Design review of the part built by this model. Coordinates are the model's own, in mm. Face numbers are marked on the shaded views. A direction names the side the tool comes from. Give positions to 0.01 mm unless a question says otherwise; leave off trailing zeros. Loops run counter-clockwise (first coordinate to the right, second up) from the corner with the lowest first, then second, coordinate; pieces in that order, holes last. Notation, with made-up numbers: (47.5, 27.5) -> (95.5, 27.5) arc R14 ccw to (95.5, 52.5) -> close; hole circle Ø9 at (55, 13). An arc over 180 degrees is marked (long way). Use a Markdown table: item, result. Add a question column.
1. For pin 1 Ø17.5 at (x, z) = (-10, 10) entering from +Y, flat-tipped, find the tip position at first contact; note if it passes through.
2. Add section C-C (z = 32.5). State the section outline as (x, y) points (1 decimal), and give its area (3 significant figures).
3. Add section D-D (y = -3). State the section outline as (x, z) points (3 decimals), and give its area (3 significant figures).
4. For the marked faces 1 and 2, list the 3-axis set-ups (+Z, -Z, +X, -X, +Y, -Y) from which the entire face can be reached by the end or side of a thin tool; tool diameter is ignored.
5. Add section B-B (y = 11). State the section outline as (x, z) points (3 decimals).
6. Add section A-A (z = 17.5). State the section outline as (x, y) points (1 decimal), and give its area (3 significant figures).
7. To check wall thickness, follow line 1 (X direction, y = -10, z = 21) (3 decimals); line 2 (Y direction, x = -28.85, z = 17.5); line 3 (Y direction, x = 27.5, z = 16). State the ranges of each line that lie inside material, in increasing order.
8. Draft analysis for pull direction X (two halves, no side actions). For the marked faces 3, 4, 5 and 6, state which applies: pulls with the +X half, pulls with the -X half, needs draft (parallel to the pull), parting line crosses it, or undercut.
```python
from build123d import *

# Parameters (mm, degrees)
SKETCH1_W           = 61.65
SKETCH1_H           = 31.375
BOSS_EXTRUDE1_DEPTH = 35
SKETCH2_W           = 51.65
SKETCH2_H           = 26.375
CUT_EXTRUDE1_DEPTH  = 50.206486171
SKETCH3_R           = 2.75
CUT_EXTRUDE2_DEPTH  = 73.607300984


with BuildPart() as part:
    # Sketch1 → Boss-Extrude1 (new body)
    with BuildSketch(Plane.XY):
        Rectangle(SKETCH1_W, SKETCH1_H)
    extrude(amount=BOSS_EXTRUDE1_DEPTH)

    # Sketch2 → Cut-Extrude1 (cut, through all)
    with BuildSketch(Plane(origin=(0, 0, 0), x_dir=(-1, 0, 0), z_dir=(0, 0, -1))):
        with Locations((0, 2.5)):
            Rectangle(SKETCH2_W, SKETCH2_H)
    extrude(amount=-CUT_EXTRUDE1_DEPTH, mode=Mode.SUBTRACT)

    # Sketch3 → Cut-Extrude2 (cut, through all)
    with BuildSketch(Plane(origin=(30.825, 0, 0), x_dir=(0, 0, -1), z_dir=(1, 0, 0))):
        with Locations((-17.5, -1.8125)):
            Circle(SKETCH3_R)
    extrude(amount=-CUT_EXTRUDE2_DEPTH, mode=Mode.SUBTRACT)


solid = part.part
```
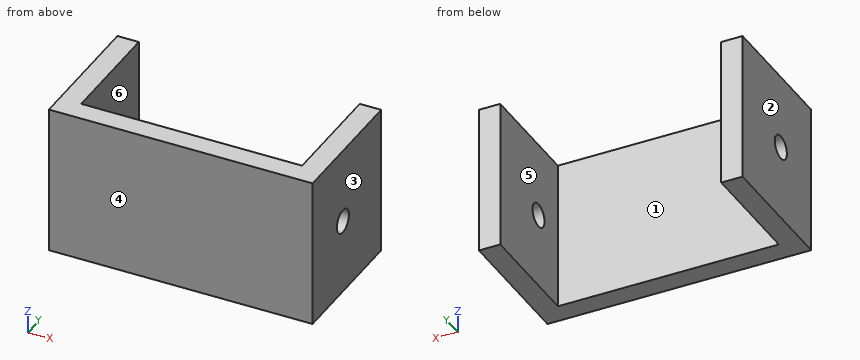
Taken from the geometry:
| question | item | result |
|---|---|---|
| 1 | pin 1 | stops at y = -10.69 |
| 2 | outline | (-30.8, -15.7) -> (30.8, -15.7) -> (30.8, 15.7) -> (25.8, 15.7) -> (25.8, -10.7) -> (-25.8, -10.7) -> (-25.8, 15.7) -> (-30.8, 15.7) -> close |
| 2 | area | 572 mm^2 |
| 3 | outline | (-30.825, 0) -> (-25.825, 0) -> (-25.825, 15.02) -> (-30.825, 15.02) -> close; (-30.825, 19.98) -> (-25.825, 19.98) -> (-25.825, 35) -> (-30.825, 35) -> close; (25.825, 0) -> (30.825, 0) -> (30.825, 15.02) -> (25.825, 15.02) -> close; (25.825, 19.98) -> (30.825, 19.98) -> (30.825, 35) -> (25.825, 35) -> close |
| 3 | area | 300 mm^2 |
| 4 | face 1 | +Z, -Z, +Y |
| 4 | face 2 | +Z, -Z, -X, +Y, -Y |
| 5 | outline | (-30.825, 0) -> (-25.825, 0) -> (-25.825, 35) -> (-30.825, 35) -> close; (25.825, 0) -> (30.825, 0) -> (30.825, 35) -> (25.825, 35) -> close |
| 6 | outline | (-30.8, -15.7) -> (30.8, -15.7) -> (30.8, -4.6) -> (25.8, -4.6) -> (25.8, -10.7) -> (-25.8, -10.7) -> (-25.8, -4.6) -> (-30.8, -4.6) -> close; (-30.8, 0.9) -> (-25.8, 0.9) -> (-25.8, 15.7) -> (-30.8, 15.7) -> close; (25.8, 0.9) -> (30.8, 0.9) -> (30.8, 15.7) -> (25.8, 15.7) -> close |
| 6 | area | 517 mm^2 |
| 7 | line 1 | x = -30.825 to -25.825, 25.825 to 30.825 |
| 7 | line 2 | y = -15.69 to -4.56, 0.94 to 15.69 |
| 7 | line 3 | y = -15.69 to -4.12, 0.49 to 15.69 |
| 8 | face 3 | pulls with the +X half |
| 8 | face 4 | needs draft |
| 8 | face 5 | undercut |
| 8 | face 6 | undercut |
